Check sheet for the drawn part. Datum: minimum x, y, z corner. Units: mm. A direction names the side the tool comes from. Coordinates: 2 decimals unless noted, no trailing zeros. Order: outer loops, then holes, each group sorted by start corner. A loop starts at its lowest first (then second) coordinate and runs counter-clockwise, first axis right, second up.
1. Thickness scan on line 1 (Y direction, x = 28, z = 2); line 2 (Y direction, x = 38, z = 2.5) (1 decimal); line 3 (X direction, y = 10.5, z = 1.5). Record the ranges inside material, lowest first.
2. Cross-section at C-C (x = 8). Enter the section's corners in (y, z) (1 decimal).
3. Cross-section at A-A (x = 28). Enter the section's corners in (y, z), then the cut area to 3 significant figures.
4. Cross-section at B-B (y = 28). Enter the section's corners in (x, z).
5. Cross-section at D-D (z = 7.25). Enter the section's corners in (x, y).
6. Gauge pin test, flat ends, axial feed: pin 1 Ø1.5 at (x, z) = (39, 2.5) entering from +Y; pin 2 Ø1 at (y, z) = (46, 4) entering from +X. Record the tip position at first contact, or that the pin passes through.
7. Draft check along Y on the marked faces 1, 2 and 3. Enter one of: released by +Y, released by -Y, zero draft, split by the parting line, or undercut.
8. Set-up check for the marked faces 4 and 5: record each of +Z, -Z, +X, -X, +Y, -Y from which the full face is reachable in a straight line by a thin tool's end or side.
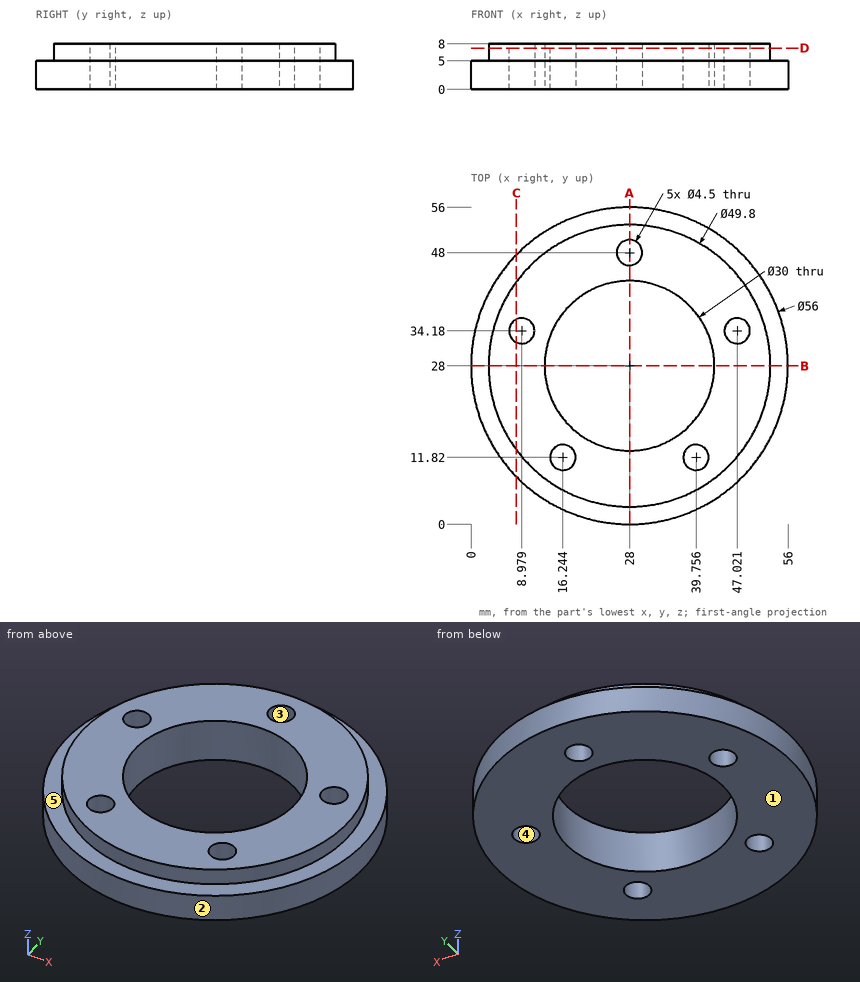
Data:
1. line 1: y = 0 to 13, 43 to 45.75, 50.25 to 56
1. line 2: y = 1.8 to 10.4, 13.2 to 16.8, 39.2 to 54.2
1. line 3: x = 6.14 to 14.42, 18.07 to 37.93, 41.58 to 49.86
2. outline: (8.4, 0) - (32.2, 0) - (32.2, 8) - (13.2, 8) - (13.2, 5) - (8.4, 5) - close; (36.2, 0) - (47.6, 0) - (47.6, 5) - (42.8, 5) - (42.8, 8) - (36.2, 8) - close
3. outline: (0, 0) - (13, 0) - (13, 8) - (3.1, 8) - (3.1, 5) - (0, 5) - close; (43, 0) - (45.75, 0) - (45.75, 8) - (43, 8) - close; (50.25, 0) - (56, 0) - (56, 5) - (52.9, 5) - (52.9, 8) - (50.25, 8) - close
3. area: 153 mm2
4. outline: (0, 0) - (13, 0) - (13, 8) - (3.1, 8) - (3.1, 5) - (0, 5) - close; (43, 0) - (56, 0) - (56, 5) - (52.9, 5) - (52.9, 8) - (43, 8) - close
5. outline: circle Ø49.8 at (28, 28); hole circle Ø4.5 at (8.98, 34.18); hole circle Ø30 at (28, 28); hole circle Ø4.5 at (16.24, 11.82); hole circle Ø4.5 at (28, 48); hole circle Ø4.5 at (39.76, 11.82); hole circle Ø4.5 at (47.02, 34.18)
6. pin 1: stops at y = 54.06
6. pin 2: stops at x = 49.86
7. face 1: zero draft
7. face 2: split by the parting line
7. face 3: undercut
8. face 4: +Z, -Z
8. face 5: +Z
